Input: dimensioned drawing with shaded views. Units: mm. Origin: part minimum x, y, z. A direction names the side the tool comes from. Give positions to 0.01 mm unless a question says otherwise; leave off trailing zeros. Order: outer loops, then holes, each group sorted by start corner. A loop starts at its lowest first (then second) coordinate and runs counter-clockwise, first axis right, second up.
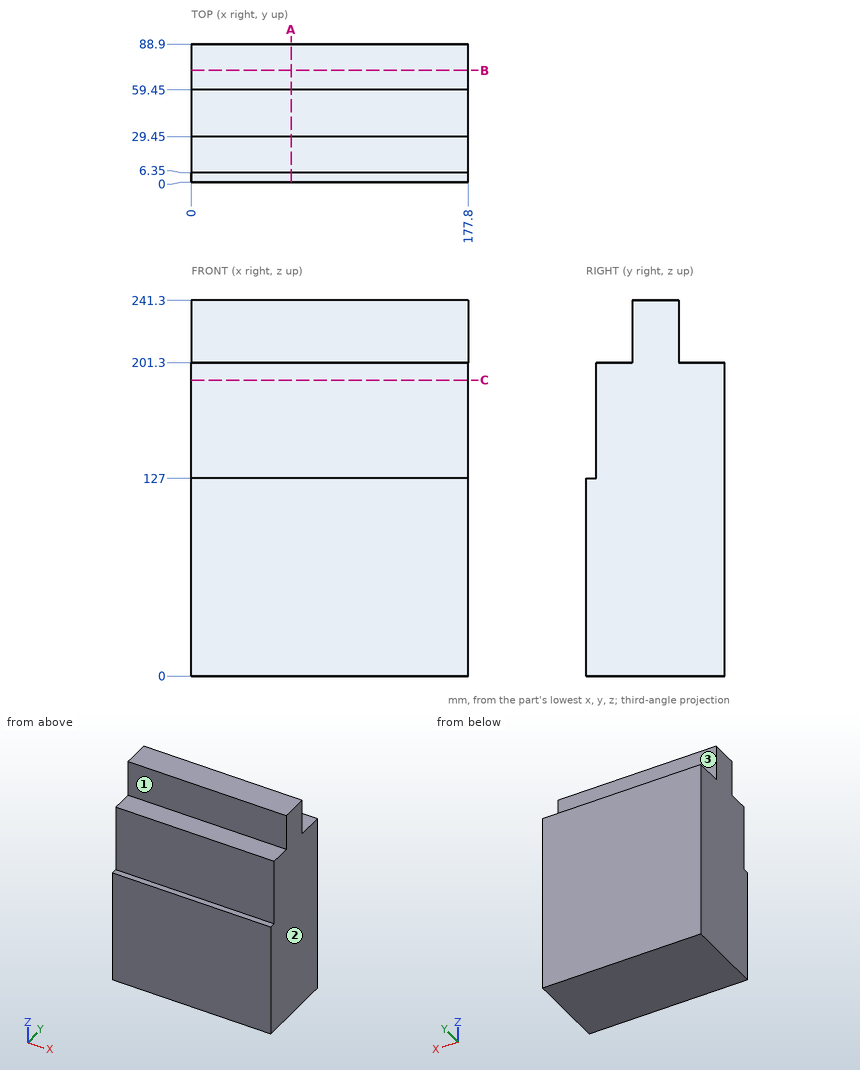
1) Section query B-B, the plane y = 72. Return the cut outline in (x, z).
Report:
outline: (0, 0) - (177.8, 0) - (177.8, 201.3) - (0, 201.3) - close
2) Reachability of the marked faces 1, 2 and 3 from +Z, -Z, +X, -X, +Y, -Y: full face, straight path, thin tool, end or side. Return the list, or none.
Report:
face 1: +Z, +X, -X, -Y
face 2: +Z, -Z, +X, +Y, -Y
face 3: +Z, +X, -X, +Y
3) Section query C-C, the plane z = 190. Return the cut outline in (x, y).
Report:
outline: (0, 6.35) - (177.8, 6.35) - (177.8, 88.9) - (0, 88.9) - close
4) Pin query (flat end, axial travel): pin 1 (12 mm diameter, centred on y = 23.5, z = 173.5, fed in from -X); pin 2 (14.5 mm diameter, centred on x = 102.5, y = 71, fed in from +Z); pin 3 (12 mm diameter, centred on x = 46.5, z = 225, fed in from -Y); pin 4 (1.9 mm diameter, centred on x = 107, y = 3, fed in from +Z). Return the tip coordinate at first contact, or that it passes through.
Report:
pin 1: stops at x = 0
pin 2: stops at z = 201.3
pin 3: stops at y = 29.45
pin 4: stops at z = 127
5) Material intervals for L1, parallel to Z at x = 115, y = 22; L2, parallel to Y at x = 13.5, z = 217.5; L3, parallel to Y at x = 94, z = 180, sorted ascending.
Report:
L1: z = 0 to 201.3
L2: y = 29.45 to 59.45
L3: y = 6.35 to 88.9
6) Section query A-A, the plane x = 64. Return the cut outline in (y, z).
Report:
outline: (0, 0) - (88.9, 0) - (88.9, 201.3) - (59.45, 201.3) - (59.45, 241.3) - (29.45, 241.3) - (29.45, 201.3) - (6.35, 201.3) - (6.35, 127) - (0, 127) - close
